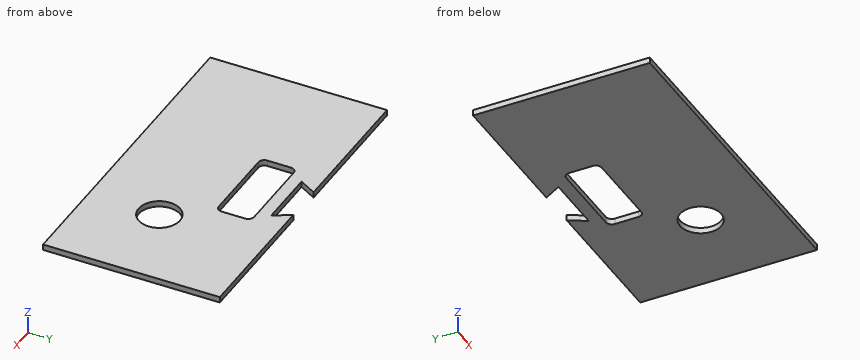
from build123d import *

# Parameters (mm, degrees)
SKETCH1_W               = 55
SKETCH1_H               = 30
BOSS_EXTRUDE1_DEPTH     = 1
CUT_EXTRUDE1_DEPTH      = 32.340867888
CUT_EXTRUDE1_DEPTH_BACK = 32.340867888
SKETCH2_R               = 3.5
SKETCH2_W               = 15
SKETCH2_H               = 6
FILLET1_R               = 1


with BuildPart() as part:
    # Sketch1 → Boss-Extrude1 (new body)
    with BuildSketch(Plane.XY):
        Rectangle(SKETCH1_W, SKETCH1_H)
    extrude(amount=BOSS_EXTRUDE1_DEPTH)

    # Sketch2 → Cut-Extrude1 (cut, two sides: drawn at the far end of the back side and taken through both)
    with BuildSketch(Plane.XY.offset(1).offset(-CUT_EXTRUDE1_DEPTH_BACK)):
        with Locations((12.5, -3)):
            Circle(SKETCH2_R)
        with Locations((0, 7)):
            Rectangle(SKETCH2_W, SKETCH2_H)
        Polygon((0, 20.773502692), (-5, 12.113248654), (5, 12.113248654), align=None)
    extrude(amount=CUT_EXTRUDE1_DEPTH + CUT_EXTRUDE1_DEPTH_BACK, mode=Mode.SUBTRACT)

    # Fillet1
    fillet1_edges = [part.edges().sort_by_distance(p)[0] for p in [
        (-7.5, 4, 0.5),
        (-7.5, 10, 0.5),
        (7.5, 10, 0.5),
        (7.5, 4, 0.5),
    ]]
    fillet(fillet1_edges, radius=FILLET1_R)


solid = part.part
Source: CAD feature listing. Evaluate the final solid. Frame: model axes, mm. Round coordinates to 2 decimals unless told otherwise and drop trailing zeros. Loops run counter-clockwise (first coordinate to the right, second up) from the corner with the lowest first, then second, coordinate; pieces in that order, holes last. Notation, with made-up numbers: (59.5, 74) - (89.5, 74) arc R24 cw to (89.5, 113) - close; hole circle Ø3 at (41.25, 29). An arc over 180 degrees is marked (long way). Write item = value, one per line. Start each with the question number.
(1) Section query B-B, the plane z = 0.8. Output: boundary loops of the cut face in (x, y).
(2) Pin query (flat end, axial travel): pin 1 (4 mm diameter, centred on x = 12.5, y = -3, fed in from +Z); pin 2 (1.5 mm diameter, centred on x = -21, y = 8.5, fed in from -Z); pin 3 (0.5 mm diameter, centred on x = -1, z = 0.5, fed in from +Y). Return the tip coordinate at first contact, or that it passes through.
(3) Ray query, line 1 along Y through (x, z) = (-0.5, 0.75); line 2 along X through (y, z) = (6, 0.7); line 3 along Y through (x, z) = (12.5, 0.65). Return the intervals inside material, ascending. Write a range as from..to.
(4) Section query A-A, the plane y = -3. Output: boundary loops of the cut face in (x, z).
(5) Section query C-C, the plane x = 12.5. Output: boundary loops of the cut face in (y, z), plus the area to 3 significant figures.
Conclusion:
q1.outline = (-27.5, -15) - (27.5, -15) - (27.5, 15) - (3.33, 15) - (5, 12.11) - (-5, 12.11) - (-3.33, 15) - (-27.5, 15) - close; hole (-7.5, 5) arc R1 ccw to (-6.5, 4) - (6.5, 4) arc R1 ccw to (7.5, 5) - (7.5, 9) arc R1 ccw to (6.5, 10) - (-6.5, 10) arc R1 ccw to (-7.5, 9) - close; hole circle Ø7 at (12.5, -3)
q2.pin_1 = through
q2.pin_2 = 0
q2.pin_3 = 12.11
q3.line_1 = -15..4, 10..12.11
q3.line_2 = -27.5..-7.5, 7.5..27.5
q3.line_3 = -15..-6.5, 0.5..15
q4.outline = (-27.5, 0) - (9, 0) - (9, 1) - (-27.5, 1) - close; (16, 0) - (27.5, 0) - (27.5, 1) - (16, 1) - close
q5.outline = (-15, 0) - (-6.5, 0) - (-6.5, 1) - (-15, 1) - close; (0.5, 0) - (15, 0) - (15, 1) - (0.5, 1) - close
q5.area = 23.0 mm2
